from build123d import *

# Parameters (mm, degrees)
SKETCH_2_W          = 23.064561435
SKETCH_2_H          = 26
SKETCH_2_R          = 1.1
EXTRUDE_1_DEPTH     = 14.5
SKETCH_3_R          = 33
CUT_EXTRUDE_1_DEPTH = 11.6
SKETCH_4_R          = 3.5
CUT_EXTRUDE_2_DEPTH = 54.268776032
SKETCH_5_W          = 15.2
SKETCH_5_H          = 29
CUT_EXTRUDE_3_DEPTH = 4
FILLET_1_R          = 3
SKETCH_6_R          = 0.9
CUT_EXTRUDE_4_DEPTH = 28.252660471
CHAMFER_1_SIZE      = 1
SKETCH_7_R          = 1.8
CUT_EXTRUDE_5_DEPTH = 1


with BuildPart() as part:
    # Эскиз2 → Бобышка-Вытянуть1 (new, symmetric)
    with BuildSketch(Plane(origin=(0, 0, 0), x_dir=(1, 0, 0), z_dir=(0, 1, 0))):
        with Locations((31.217719282, 0)):
            Rectangle(SKETCH_2_W, SKETCH_2_H)
        with Locations(Location((23.685438565, 8, 0), (0, 0, 90))):
            Circle(SKETCH_2_R, mode=Mode.SUBTRACT)
        with Locations(Location((23.685438565, -8, 0), (0, 0, 90))):
            Circle(SKETCH_2_R, mode=Mode.SUBTRACT)
    extrude(amount=EXTRUDE_1_DEPTH, both=True)

    # Эскиз3 → Вырез-Вытянуть1 (cut, symmetric)
    with BuildSketch(Plane(origin=(0, 0, 0), x_dir=(1, 0, 0), z_dir=(0, 1, 0))):
        Circle(SKETCH_3_R)
    extrude(amount=CUT_EXTRUDE_1_DEPTH, both=True, mode=Mode.SUBTRACT)

    # Эскиз4 → Вырез-Вытянуть2 (cut, through all)
    with BuildSketch(Plane(origin=(0, 14.5, 0), x_dir=(1, 0, 0), z_dir=(0, 1, 0))):
        with Locations((25, 0)):
            Circle(SKETCH_4_R)
        with BuildLine():
            ThreePointArc((25, -3.5), (21.5, 0), (25, 3.5))
            Line((25, 3.5), (19.685438565, 3.5))
            Line((19.685438565, 3.5), (19.685438565, -3.5))
            Line((19.685438565, -3.5), (25, -3.5))
        make_face()
    extrude(amount=-CUT_EXTRUDE_2_DEPTH, mode=Mode.SUBTRACT)

    # Эскиз5 → Вырез-Вытянуть3 (cut)
    with BuildSketch(Plane(origin=(42.75, 0, 0), x_dir=(0, 0, -1), z_dir=(1, 0, 0))):
        Rectangle(SKETCH_5_W, SKETCH_5_H)
    extrude(amount=-CUT_EXTRUDE_3_DEPTH, mode=Mode.SUBTRACT)

    # Скругление1
    fillet_1_edges = [part.edges().sort_by_distance(p)[0] for p in [
        (19.685438565, -13.05, 13),
        (19.685438565, -13.05, -13),
        (19.685438565, 13.05, 3.5),
        (19.685438565, 13.05, -3.5),
        (19.685438565, -13.05, 3.5),
        (19.685438565, -13.05, -3.5),
        (42.75, 0, 13),
        (19.685438565, 13.05, 13),
        (19.685438565, 13.05, -13),
        (42.75, 0, -13),
    ]]
    fillet(fillet_1_edges, radius=FILLET_1_R)

    # Эскиз6 → Вырез-Вытянуть4 (cut, through all)
    with BuildSketch(Plane(origin=(38.75, 0, 0), x_dir=(0, 0, -1), z_dir=(1, 0, 0))):
        with Locations((0, 6)):
            Circle(SKETCH_6_R)
        with Locations((0, -6)):
            Circle(SKETCH_6_R)
    extrude(amount=-CUT_EXTRUDE_4_DEPTH, mode=Mode.SUBTRACT)

    # Фаска1
    chamfer_1_edges = [part.edges().sort_by_distance(p)[0] for p in [
        (20.564118221, 14.5, 12.121320344),
        (20.564118221, 14.5, 4.378679656),
        (20.564118221, 14.5, -4.378679656),
        (20.564118221, 14.5, -12.121320344),
        (41.871320344, 14.5, -12.121320344),
        (28.5, -14.5, 0),
        (23.842719282, -14.5, -3.5),
        (28.5, 14.5, 0),
        (23.842719282, 14.5, -3.5),
        (42.75, -14.5, -8.8),
        (42.75, 14.5, -8.8),
        (31.217719282, 14.5, -13),
        (31.217719282, -14.5, -13),
        (42.75, -14.5, 8.8),
        (31.217719282, -14.5, 13),
        (19.685438565, -14.5, 8.25),
        (23.842719282, -14.5, 3.5),
        (19.685438565, -14.5, -8.25),
        (41.871320344, -14.5, 12.121320344),
        (20.564118221, -14.5, 12.121320344),
        (20.564118221, -14.5, 4.378679656),
        (20.564118221, -14.5, -4.378679656),
        (20.564118221, -14.5, -12.121320344),
        (41.871320344, -14.5, -12.121320344),
        (19.685438565, 14.5, -8.25),
        (23.842719282, 14.5, 3.5),
        (19.685438565, 14.5, 8.25),
        (31.217719282, 14.5, 13),
        (42.75, 14.5, 8.8),
        (41.871320344, 14.5, 12.121320344),
    ]]
    chamfer(chamfer_1_edges, length=CHAMFER_1_SIZE)

    # Эскиз7 → Вырез-Вытянуть5 (cut)
    with BuildSketch(Plane(origin=(0, 14.5, 0), x_dir=(1, 0, 0), z_dir=(0, 1, 0))):
        with Locations(Location((23.685438565, 8, 0), (0, 0, 270))):
            Circle(SKETCH_7_R)
        with Locations(Location((23.685438565, -8, 0), (0, 0, 270))):
            Circle(SKETCH_7_R)
    cut_extrude_5 = extrude(amount=-CUT_EXTRUDE_5_DEPTH, mode=Mode.SUBTRACT)

    # Зеркальное отражение1: Вырез-Вытянуть5 across plane
    add(cut_extrude_5.mirror(Plane.ZX), mode=Mode.SUBTRACT)


solid = part.part
Can you work these out from the model? Positions are in its coordinate system, mm. A direction names the side the tool comes from. Round coordinates to 2 decimals unless told otherwise and drop trailing zeros. Write each loop counter-clockwise with the first axis right and the second up, starting at its lowest first coordinate (ties: lowest second). Pieces come first, ordered by that corner, then holes. Notation, with made-up numbers: M 41,-12.75 L 61,-12.75 A23 cw 61,25.25 Z; hole C 49,7.5 d7. An arc over 180 degrees is marked long. Use a Markdown table: item, result.
Item 1: Which directions (+Z, -Z, +X, -X, +Y, -Y) give clear straight access to the entire face, cutting with the end or side of a thin tool? Please do faces 1 (the face through (41, 0, -7.6)), 2 (the face through (24, -14, 4)), 3 (the face through (21.93, 14.01, 7.61)), 4 (the face through (20.588, -12.563, -4.355)).
Found:
| item | result |
|---|---|
| face 1 | +X, +Y, -Y |
| face 2 | -X, -Y |
| face 3 | +Y |
| face 4 | -X, +Y, -Y |
Item 2: I want a section at C-C (y = -2.75). List the corners of the cut face in (x, z) for me, and give its area (3 significant figures).
Found:
| item | result |
|---|---|
| outline | M 30.33,-13 L 39.75,-13 A3 ccw 42.75,-10 L 42.75,-7.6 L 38.75,-7.6 L 38.75,7.6 L 42.75,7.6 L 42.75,10 A3 ccw 39.75,13 L 30.33,13 A33 cw Z |
| area | 212 mm2 |
Item 3: I want a section at A-A (y = 6). List the corners of the cut face in (x, z) for me.
Found:
| item | result |
|---|---|
| outline | M 30.33,-13 L 39.75,-13 A3 ccw 42.75,-10 L 42.75,-7.6 L 38.75,-7.6 L 38.75,-0.9 L 32.99,-0.9 A33 cw Z; M 30.33,13 A33 cw 32.99,0.9 L 38.75,0.9 L 38.75,7.6 L 42.75,7.6 L 42.75,10 A3 ccw 39.75,13 Z |
Item 4: We'd pull the mould along Z, two halves only. Please class faces 5 (the face through (31.3, -14, 12.5)), 6 (the face through (19.685, 13, 8)), 7 (the face through (29, -14, 0)): released by +Z, released by -Z, zero draft, split by the parting line, or undercut.
Found:
| item | result |
|---|---|
| face 5 | released by +Z |
| face 6 | zero draft |
| face 7 | undercut |
Item 5: I want a section at B-B (z = 0). List the corners of the cut face in (x, y) for me.
Found:
| item | result |
|---|---|
| outline | M 28.5,-13.5 L 29.5,-14.5 L 38.75,-14.5 L 38.75,-6.9 L 33,-6.9 L 33,-11.6 L 28.5,-11.6 Z; M 28.5,11.6 L 33,11.6 L 33,6.9 L 38.75,6.9 L 38.75,14.5 L 29.5,14.5 L 28.5,13.5 Z; M 33,-5.1 L 38.75,-5.1 L 38.75,5.1 L 33,5.1 Z |
Item 6: For pin 1 Ø4.5 at (y, z) = (0.5, -2) entering from +X; pin 2 Ø3 at (x, z) = (23.69, 8) entering from -Y; pin 3 Ø1.3 at (x, z) = (23.69, 8) entering from +Y, each with a flat end and sliding along its axis, tell me the tip position at first contact or that it passes through.
Found:
| item | result |
|---|---|
| pin 1 | stops at x = 38.75 |
| pin 2 | stops at y = -13.5 |
| pin 3 | passes through |
Item 7: I want a section at D-D (x = 31.75). List the corners of the cut face in (y, z) for me.
Found:
| item | result |
|---|---|
| outline | M -14.5,-12 L -13.5,-13 L 13.5,-13 L 14.5,-12 L 14.5,12 L 13.5,13 L -13.5,13 L -14.5,12 Z; hole M -11.6,-9 L 11.6,-9 L 11.6,9 L -11.6,9 Z |
Item 8: If I drill on line 1 along Y through (x, z) = (35.75, 0); line 2 along Y through (x, z) = (29.25, 11.5); line 3 along Z through (x, y) = (37.65, 6), over which ranges is the centre line in solid material (lowest first)? Write a range as [from, to].
Found:
| item | result |
|---|---|
| line 1 | y = [-14.5, -6.9], [-5.1, 5.1], [6.9, 14.5] |
| line 2 | y = [-14.5, -11.6], [11.6, 14.5] |
| line 3 | z = [-13, -0.9], [0.9, 13] |
